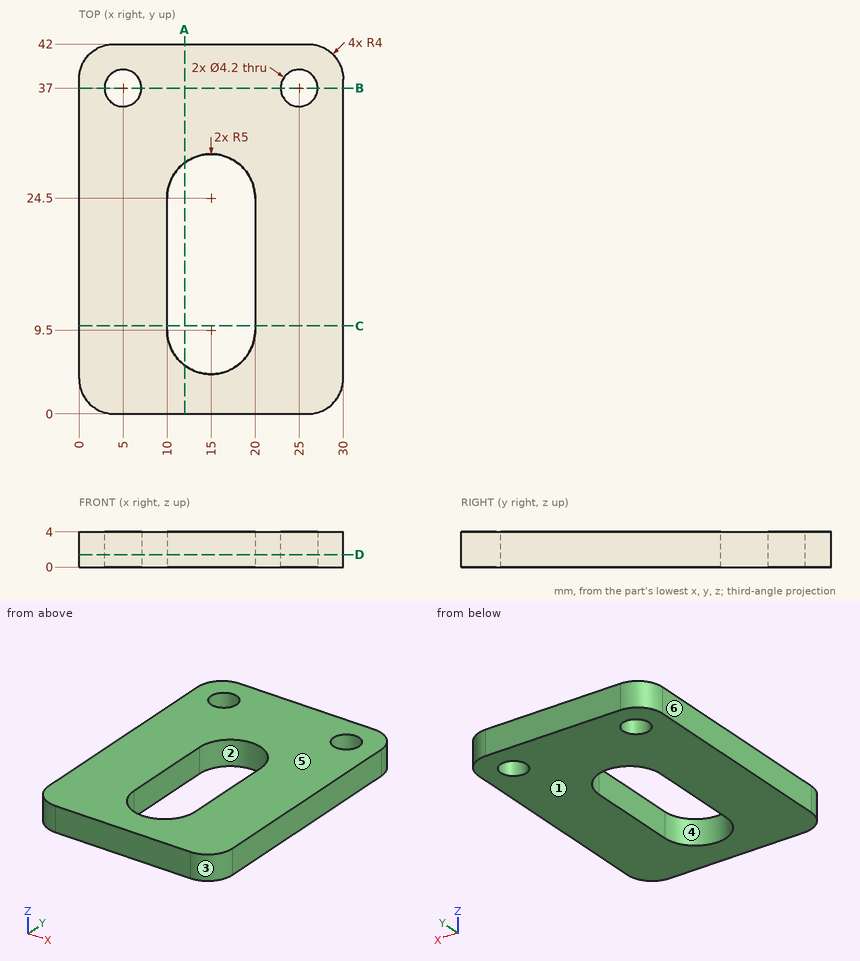
Input: dimensioned drawing with shaded views. Units: mm. Origin: part minimum x, y, z. A direction names the side the tool comes from. Round coordinates to 2 decimals unless told otherwise and drop trailing zeros. Loops run counter-clockwise (first coordinate to the right, second up) from the corner with the lowest first, then second, coordinate; pieces in that order, holes last. Notation, with made-up numbers: M 16.5,13.5 L 62.5,13.5 A11 cw 62.5,34.5 Z; hole C 73.5,42 d8. An arc over 180 degrees is marked long. One line per question, with ' | ' between items.
(1) Access query for the marked faces 1 and 2. Directions: +Z, -Z, +X, -X, +Y, -Y. A direction counts if a zero-diameter tool reaches every point of the face in a straight line with its end or side. Return the directions, or none.
Check result:
face 1: -Z, +X, -X, +Y, -Y | face 2: +Z, -Z
(2) Cut plane C-C on y = 10. Return the cut outline in (x, z).
Check result:
outline: M 0,0 L 10,0 L 10,4 L 0,4 Z; M 20,0 L 30,0 L 30,4 L 20,4 Z
(3) Pull-direction query (X, two-part tool) for the marked faces 3, 4, 5 and 6; classes: +X half, -X half, draft (parallel to the pull), parting line (faces both ways), or undercut.
Check result:
face 3: +X half | face 4: undercut | face 5: draft | face 6: -X half
(4) Cut plane D-D on z = 1.4. Return the cut outline in (x, y), plus the area to 3 significant figures.
Check result:
outline: M 0,4 A4 ccw 4,0 L 26,0 A4 ccw 30,4 L 30,38 A4 ccw 26,42 L 4,42 A4 ccw 0,38 Z; hole C 5,37 d4.2; hole M 10,9.5 A5 ccw 20,9.5 L 20,24.5 A5 ccw 10,24.5 Z; hole C 25,37 d4.2 | area: 990 mm2
(5) Cut plane A-A on x = 12. Return the cut outline in (y, z), plus the area to 3 significant figures.
Check result:
outline: M 0,0 L 5.5,0 L 5.5,4 L 0,4 Z; M 28.5,0 L 42,0 L 42,4 L 28.5,4 Z | area: 76.0 mm2
(6) Material intervals for line 1 along Y through (x, z) = (25, 1.25); line 2 along X through (y, z) = (13, 2.35); line 3 along Y through (x, z) = (25.5, 0.3), sorted ascending. Write a range as from..to.
Check result:
line 1: y = 0..34.9, 39.1..42 | line 2: x = 0..10, 20..30 | line 3: y = 0..34.96, 39.04..42
(7) Contact query for a flat-ended pin moving along its axis: P1, Ø4, axis at x = 25, y = 37, coming from the -Z side. Output: stop coordinate, or through.
Check result:
P1: passes through
(8) Cut plane B-B on y = 37. Return the cut outline in (x, z).
Check result:
outline: M 0,0 L 2.9,0 L 2.9,4 L 0,4 Z; M 7.1,0 L 22.9,0 L 22.9,4 L 7.1,4 Z; M 27.1,0 L 30,0 L 30,4 L 27.1,4 Z
